```python
from build123d import *

# Parameters (mm, degrees)
F0_W      = 43.5
F0_H      = 43.5
F3_W      = 35.5
F3_H      = 35.5
F6_R      = 1.55
F8_DEPTH  = 9.0010001
F9_DEPTH  = 9.0010001
F10_DEPTH = 2.5
F11_DEPTH = 2.5


with BuildPart() as f4:
    # F0 (on Top) → F4 section 0
    with BuildSketch(Plane.XY):
        Rectangle(F0_W, F0_H)
    # F3 (on offset) → F4 section 1
    with BuildSketch(Plane.XY.offset(9)):
        Rectangle(F3_W, F3_H)
    loft()

    # F6 (on face) → F8 (cut, through all)
    with BuildSketch(Plane.XY.offset(9)):
        with Locations((0, 7.5)):
            Circle(F6_R)
    extrude(amount=-F8_DEPTH, mode=Mode.SUBTRACT)

    # F6 (on face) → F9 (cut, through all)
    with BuildSketch(Plane.XY.offset(9)):
        with Locations((0, -7.5)):
            Circle(F6_R)
    extrude(amount=-F9_DEPTH, mode=Mode.SUBTRACT)

    # F7 (on Top) → F10 (cut)
    with BuildSketch(Plane.XY):
        Polygon((0.3239838625, -10.6008119029), (2.8473738115, -8.7698276961), (2.523389949, -5.6690157933), (-0.3239838625, -4.3991880971), (-2.8473738115, -6.2301723039), (-2.523389949, -9.3309842067), align=None)
    extrude(amount=F10_DEPTH, mode=Mode.SUBTRACT)

    # F7 (on Top) → F11 (cut)
    with BuildSketch(Plane.XY):
        Polygon((3.1175957979, 7.4755778561), (1.579948096, 10.1877060877), (-1.5376477019, 10.2121282317), (-3.1175957979, 7.5244221439), (-1.579948096, 4.8122939123), (1.5376477019, 4.7878717683), align=None)
    extrude(amount=F11_DEPTH, mode=Mode.SUBTRACT)


solid = f4.part
```
Check sheet for the modelled part. Datum: model origin and axes. Units: mm. A direction names the side the tool comes from. Coordinates: 2 decimals unless noted, no trailing zeros. Write each question's results on one line, items separated by ' | '. Start each with the question number.
1) Section check A-A (z = 8.25). Count the separate pieces of the cut face and the enclosed holes in it, and give its area (3 significant figures).
2) Material ranges on line 1 along Y through (x, z) = (0, 7); line 2 along Y through (x, z) = (0, 4); line 3 along Z through (x, y) = (0.5, -10), recorded low to high.
3) Depth check by flat-ended pin: pin 1 (3 mm diameter, centred on x = 0, y = -7.5, fed in from -Z); pin 2 (4 mm diameter, centred on x = 0, y = 7.5, fed in from -Z); pin 3 (3 mm diameter, centred on x = 15.5, z = 5, fed in from +Y); pin 4 (4 mm diameter, centred on x = -11, z = 2.5, fed in from +Y). Enter the tip coordinate at first touch or a pass-through.
4) Draft check along Y on faces 3 (the face through (0, 0, 9)), 4 (the face through (-2.688, -7.759, 1.232)). Enter one of: pulls with the +Y half, pulls with the -Y half, needs draft (parallel to the pull), parting line crosses it, or undercut.
5) Set-up check for faces 1 (the face through (1.568, -9.698, 1.232)), 2 (the face through (-0.336, -9.013, 5.796)): record each of +Z, -Z, +X, -X, +Y, -Y from which the full face is reachable in a straight line by a thin tool's end or side.
Checked values:
1) separate pieces: 1 | enclosed holes: 2 | area: 1,290 mm²
2) line 1: -18.64 to -9.05, -5.95 to 5.95, 9.05 to 18.64 | line 2: -19.97 to -9.05, -5.95 to 5.95, 9.05 to 19.97 | line 3: 2.5 to 9
3) pin 1: through | pin 2: z = 2.5 | pin 3: y = 20.19 | pin 4: y = 21.53
4) face 3: needs draft | face 4: undercut
5) face 1: -Z | face 2: +Z, -Z
